from build123d import *

# Parameters (mm, degrees)
SKETCH_1_W          = 40
SKETCH_1_H          = 9
SKETCH_1_R          = 2
EXTRUDE_1_DEPTH     = 5
SKETCH_2_W          = 0.8
SKETCH_2_H          = 1
CUT_EXTRUDE_1_DEPTH = 23.494443758


with BuildPart() as part:
    # 草圖1 → 填料-伸長1 (new body)
    with BuildSketch(Plane.XY):
        Rectangle(SKETCH_1_W, SKETCH_1_H)
        Circle(SKETCH_1_R, mode=Mode.SUBTRACT)
    extrude(amount=EXTRUDE_1_DEPTH)

    # 草圖2 → 除料-伸長1 (cut, through all)
    with BuildSketch(Plane.XZ.offset(4.5)):
        with Locations((-18.8, 4.5)):
            Rectangle(SKETCH_2_W, SKETCH_2_H)
        with Locations((-16.8, 4.5)):
            Rectangle(SKETCH_2_W, SKETCH_2_H)
        with Locations((-14.8, 4.5)):
            Rectangle(SKETCH_2_W, SKETCH_2_H)
        with Locations((-12.8, 4.5)):
            Rectangle(SKETCH_2_W, SKETCH_2_H)
        with Locations((-10.8, 4.5)):
            Rectangle(SKETCH_2_W, SKETCH_2_H)
        Polygon((-9.2, 4), (-8.4, 4), (8.4, 4), (9.2, 4), (9.2, 5), (8.4, 5), (-8.4, 5), (-9.2, 5), align=None)
        with Locations((10.8, 4.5)):
            Rectangle(SKETCH_2_W, SKETCH_2_H)
        with Locations((12.8, 4.5)):
            Rectangle(SKETCH_2_W, SKETCH_2_H)
        with Locations((14.8, 4.5)):
            Rectangle(SKETCH_2_W, SKETCH_2_H)
        with Locations((16.8, 4.5)):
            Rectangle(SKETCH_2_W, SKETCH_2_H)
        with Locations((18.8, 4.5)):
            Rectangle(SKETCH_2_W, SKETCH_2_H)
    extrude(amount=-CUT_EXTRUDE_1_DEPTH, mode=Mode.SUBTRACT)


solid = part.part
Design review of the part built by this model. Coordinates are the model's own, in mm. A direction names the side the tool comes from. Round coordinates to 2 decimals unless told otherwise and drop trailing zeros. Write each loop counter-clockwise with the first axis right and the second up, starting at its lowest first coordinate (ties: lowest second). Pieces come first, ordered by that corner, then holes. Notation, with made-up numbers: (-8.5, -18.5) - (25.5, -18.5) arc R31 ccw to (25.5, 15.5) - close; hole circle Ø5 at (60.5, 7). An arc over 180 degrees is marked (long way). Use a Markdown table: item, result. Add a question column.
1. Mouldability with a two-part tool opening along X and no side actions: class faces 1 (the face through (12.4, -0.1, 4.5)), 2 (the face through (-14.4, -0.1, 4.5)), 3 (the face through (0, 4.5, 2)) as +X half, -X half, draft (parallel to the pull), parting line (faces both ways), or undercut.
2. For faces 4 (the face through (16.4, -0.1, 4.5)), 5 (the face through (-14, 0, 5)), list the 3-axis set-ups (+Z, -Z, +X, -X, +Y, -Y) from which the entire face can be reached by the end or side of a thin tool; tool diameter is ignored.
3. We need section C-C (x = 8). State the section outline as (y, z) points.
4. Wall thickness on probe 1 along X at (y, z) = (0, 1.35); probe 2 along Y at (x, z) = (0, 0.8); probe 3 along Z at (x, y) = (15, -2): over which ranges is each line inside the solid? List them lowest first.
5. We need section B-B (z = 0.4). State the section outline as (x, y) points, then the cut area to 3 significant figures.
6. We need section A-A (x = 0). State the section outline as (y, z) points, then the cut area to 3 significant figures.
Output:
| question | item | result |
|---|---|---|
| 1 | face 1 | undercut |
| 1 | face 2 | undercut |
| 1 | face 3 | draft |
| 2 | face 4 | +Z, +Y, -Y |
| 2 | face 5 | +Z, +X, -X, +Y, -Y |
| 3 | outline | (-4.5, 0) - (4.5, 0) - (4.5, 4) - (-4.5, 4) - close |
| 4 | probe 1 | x = -20 to -2, 2 to 20 |
| 4 | probe 2 | y = -4.5 to -2, 2 to 4.5 |
| 4 | probe 3 | z = 0 to 4 |
| 5 | outline | (-20, -4.5) - (20, -4.5) - (20, 4.5) - (-20, 4.5) - close; hole circle Ø4 at (0, 0) |
| 5 | area | 347 mm2 |
| 6 | outline | (-4.5, 0) - (-2, 0) - (-2, 4) - (-4.5, 4) - close; (2, 0) - (4.5, 0) - (4.5, 4) - (2, 4) - close |
| 6 | area | 20.0 mm2 |
